The model under review builds one solid part; all positions refer to its coordinate system, in mm. Face numbers are marked on the shaded views. A direction names the side the tool comes from. Round coordinates to 2 decimals unless told otherwise and drop trailing zeros. Write each loop counter-clockwise with the first axis right and the second up, starting at its lowest first coordinate (ties: lowest second). Pieces come first, ordered by that corner, then holes.
Item 1: To check wall thickness, follow L1, parallel to X at y = 0, z = 10.5; L2, parallel to Y at x = 0, z = 3.75. State the ranges of each line that lie inside material, in increasing order.
Item 2: Draft analysis for pull direction Y (two halves, no side actions). For the marked faces 6, 7 and 8, state which applies: +Y half, -Y half, draft (parallel to the pull), parting line (faces both ways), or undercut.
Item 3: Add section A-A (z = 27.5). Give the boundary of the cut face in (x, y), plus the area to 3 significant figures.
Item 4: Machinability: for the marked faces 1, 2, 3, 4 and 5, which of the approach directions +Z, -Z, +X, -X, +Y, -Y give a long, thin tool a straight path to every point of the face, cutting with its end or side? Answer none if there is none.
Item 5: Clearance check with flat-ended pins moving along their axes: pin 1 Ø1.5 at (x, y) = (3.5, 7) entering from +Z; pin 2 Ø1.5 at (x, y) = (4.5, -8.5) entering from +Z; pin 3 Ø12.5 at (x, z) = (2, 19.5) entering from +Y; pin 4 Ø10 at (y, z) = (2, 18.5) entering from +X. State where each tip first meets the part, or that it passes through.
Autodesk Fusion 360 part; units mm, degrees
sketch "Sketch1" plane through (0, 0, 0) normal (0, 0, 1) x (1, 0, 0)
  circle A0 centre (0, 0) radius 30
  line L0 (15, 15) -> (-15, 15)
  line L1 (-15, 15) -> (-15, -15)
  line L2 (-15, -15) -> (15, -15)
  line L3 (15, -15) -> (15, 15)
  line L4 (15, 15) -> (-15, -15) construction
  line L5 (-15, 15) -> (15, -15) construction
  dimension "d1" = 60
  dimension "d2" = 30
  dimension "d3" = 30
extrude "Extrude1" add sketch "Sketch1" along normal blind 10
extrude "Extrude3" add sketch "Sketch1" along normal blind 30 contours L0 L1 L2 L3
sketch "Sketch3" plane through (0, 0, 30) normal (0, 0, 1) x (-1, 0, 0)
  line L0 (5.7735, -10) -> (11.547, 0)
  line L1 (11.547, 0) -> (5.7735, 10)
  line L2 (5.7735, 10) -> (-5.7735, 10)
  line L3 (-5.7735, 10) -> (-11.547, 0)
  line L4 (-11.547, 0) -> (-5.7735, -10)
  line L5 (-5.7735, -10) -> (5.7735, -10)
  dimension "d11" = 20
  dimension "d12" = 23.094
extrude "Extrude4" cut sketch "Sketch3" against normal blind 15
sketch "Sketch4" plane through (0, 0, 30) normal (0, 0, 1) x (-1, 0, 0)
  circle A0 centre (0, 0) radius 10
  line L0 (-5.7735, -10) -> (-11.547, 0)
extrude "Extrude5" cut sketch "Sketch4" against normal blind 55
fillet "Fillet1" radius 2 1 edges at (-27.9698, -10.8485, 10)
chamfer "Chamfer1" distance 2 angle 45 4 edges at (-15, -15, 20) (-15, 15, 20) (15, 15, 20) (15, -15, 20)
sketch "Sketch2" plane through (0, 0, 30) normal (0, 0, 1) x (-1, 0, 0)
  line L0 (0.7735, -12.8868) -> (11.547, -5.7735)
  line L1 (11.547, -5.7735) -> (10.7735, 7.1132)
  line L2 (10.7735, 7.1132) -> (-0.7735, 12.8868)
  line L3 (-0.7735, 12.8868) -> (-11.547, 5.7735)
  line L4 (-11.547, 5.7735) -> (-10.7735, -7.1132)
  line L5 (-10.7735, -7.1132) -> (0.7735, -12.8868)
extrude "Extrude2" [suppressed]
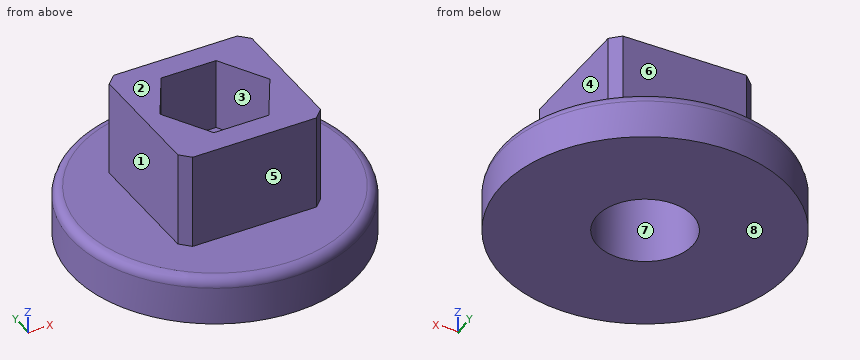
Numbers:
1. L1: x = -15 to -10, 10 to 15
1. L2: y = -30 to -10, 10 to 30
2. face 6: +Y half
2. face 7: undercut
2. face 8: draft
3. outline: (-15, -13) - (-13, -15) - (13, -15) - (15, -13) - (15, 13) - (13, 15) - (-13, 15) - (-15, 13) - close; hole (-11.55, 0) - (-5.77, -10) - (5.77, -10) - (11.55, 0) - (5.77, 10) - (-5.77, 10) - close
3. area: 546 mm2
4. face 1: +Z, -X, +Y, -Y
4. face 2: +Z, +X, -X, +Y, -Y
4. face 3: +Z
4. face 4: +Z, +X, +Y, -Y
4. face 5: +Z, +X, -X, -Y
5. pin 1: passes through
5. pin 2: stops at z = 15
5. pin 3: stops at y = 15
5. pin 4: stops at x = 15
